Geometry check sheet. Reference: drawing and pictorial views, mm from the part's lowest x, y, z. Round coordinates to 2 decimals unless told otherwise and drop trailing zeros. Order: outer loops, then holes, each group sorted by start corner. A loop starts at its lowest first (then second) coordinate and runs counter-clockwise, first axis right, second up.
Q1. Cross-section at A-A on x = 1.5. Record the cut outline in (y, z).
Q2. Depth check by flat-ended pin: P1, Ø5, axis at x = 16, z = 4, coming from the -Y side; P2, Ø3, axis at x = 15.5, y = 1.5, coming from the -Z side (1 decimal). Enter the tip coordinate at first touch or a pass-through.
Q3. Scan lines: probe 1 along X at (y, z) = (0.5, 5.5) (1 decimal); probe 2 along X at (y, z) = (7, 8.75) (1 decimal); probe 3 along Z at (x, y) = (22.5, 5) (1 decimal). Record each from-to range of solid material in increasing order.
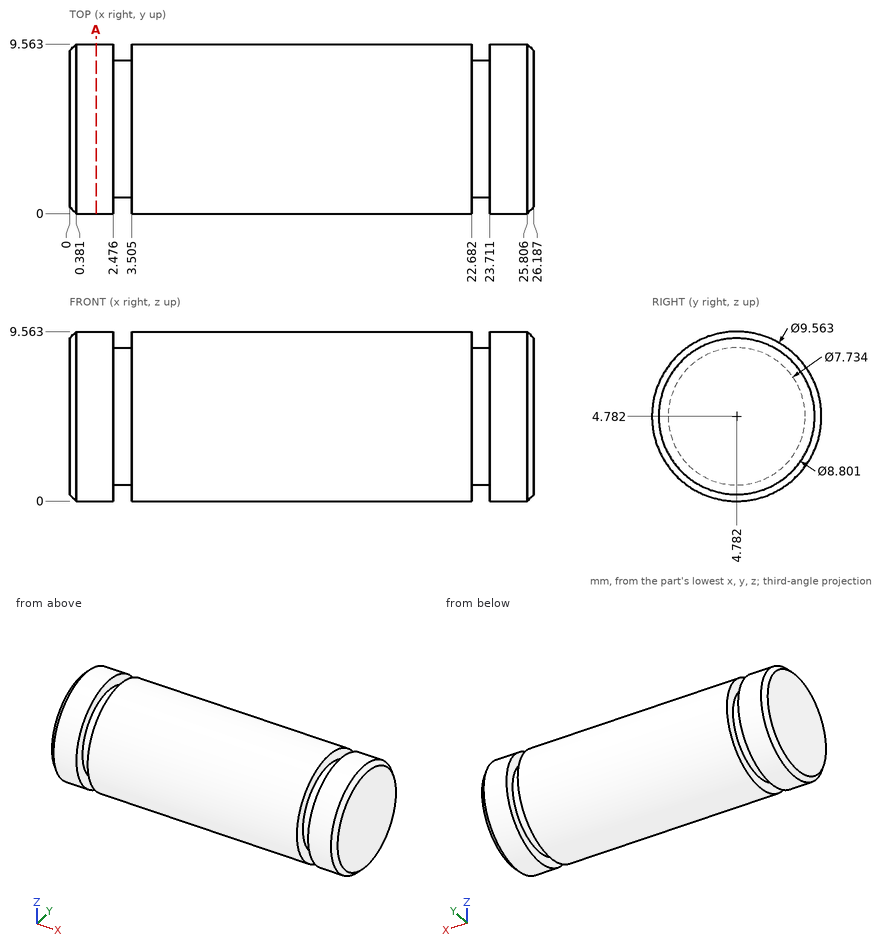
Results found:
1. outline: circle Ø9.56 at (4.78, 4.78)
2. P1: stops at y = 0
2. P2: stops at z = 0.3
3. probe 1: x = 0 to 2.5, 3.5 to 22.7, 23.7 to 26.2
3. probe 2: x = 0.1 to 2.5, 3.5 to 22.7, 23.7 to 26
3. probe 3: z = 0 to 9.6
